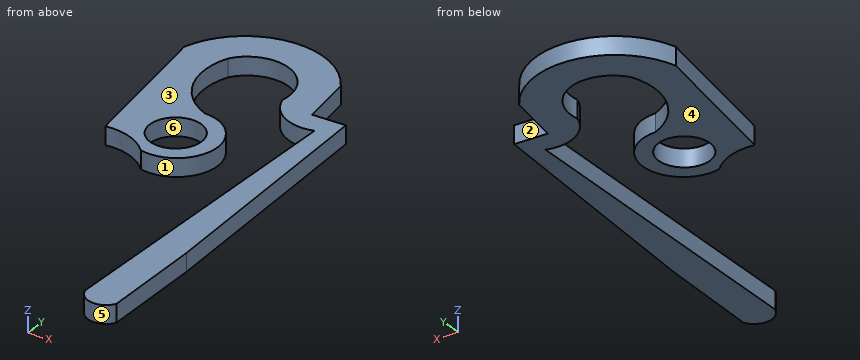
```python
from build123d import *

# Parameters (mm, degrees)
SKETCH1_R           = 1.27
BOSS_EXTRUDE1_DEPTH = 0.889


with BuildPart() as part:
    # Sketch1 → Boss-Extrude1 (new body)
    with BuildSketch(Plane.XY):
        with BuildLine():
            Line((-4.521957117, 7.997023921), (-3.500640843, 0.843746079))
            ThreePointArc((-3.500640843, 0.843746079), (-2.247752793, 0.722417864), (-1.189432305, 0.040943912))
            ThreePointArc((-1.189432305, 0.040943912), (1.231506645, 1.78476828), (-0.761885285, 4.004736172))
            ThreePointArc((-0.761885285, 4.004736172), (-2.523808067, 5.75027928), (-2.507561872, 8.230406029))
            ThreePointArc((-2.507561872, 8.230406029), (-0.008086329, 8.999486055), (1.23243455, 6.697319679))
            ThreePointArc((1.23243455, 6.697319679), (2.203084663, 5.504138097), (3.734868812, 5.364562852))
            Line((3.734868812, 5.364562852), (3.409647754, -10.616831622))
            ThreePointArc((3.409647754, -10.616831622), (4.172569321, -11.302719528), (5.081281403, -10.826553706))
            Line((5.081281403, -10.826553706), (5.081281403, -5.788347659))
            Line((5.081281403, -5.788347659), (4.536062194, 6.463867416))
            Line((4.536062194, 6.463867416), (2.910345816, 6.391523616))
            Line((2.910345816, 6.391523616), (2.548786355, 8.982410145))
            ThreePointArc((2.548786355, 8.982410145), (-1.304965957, 10.774290658), (-4.521957117, 7.997023921))
        make_face()
        with Locations((-0.822961988, 2.012924292)):
            Circle(SKETCH1_R, mode=Mode.SUBTRACT)
    extrude(amount=BOSS_EXTRUDE1_DEPTH)


solid = part.part
```
Input: part model. Units: mm. Frame: model coordinates. Face numbers are marked on the shaded views. A direction names the side the tool comes from. Round coordinates to 2 decimals unless told otherwise and drop trailing zeros. Loops run counter-clockwise (first coordinate to the right, second up) from the corner with the lowest first, then second, coordinate; pieces in that order, holes last. Notation, with made-up numbers: M -13,0.5 L 43,0.5 A23 ccw 43,12.5 Z; hole C 8.25,15 d9. An arc over 180 degrees is marked long. Answer in a Markdown table with one row per item. Add a question column.
1. Ray query, probe 1 along Y at (x, z) = (-1.5, 0.25); probe 2 along Y at (x, z) = (-1.25, 0.05); probe 3 along X at (y, z) = (2, 0.75). Return the intervals inside material, ascending.
2. Section A-A (y = 4.5). Output: boundary loops of the cut face in (x, z), and give its area (3 significant figures).
3. Set-up query: the marked faces 1, 2 and 3. Return all of +Z, -Z, +X, -X, +Y, -Y with unobstructed straight access to the full face (end or side cutting, diameter ignored); none if empty.
4. Section B-B (z = 0.45). Output: boundary loops of the cut face in (x, y).
5. Mould query, pull axis X, two halves, no side actions, for the marked faces 4, 5 and 6. Classes: released by +X, released by -X, zero draft, split by the parting line, or undercut.
6. Section D-D (y = -6.75). Output: boundary loops of the cut face in (x, z), and give its area (3 significant figures).
7. Section C-C (x = -0.25). Output: boundary loops of the cut face in (y, z), and give its area (3 significant figures).
Values follow:
| question | item | result |
|---|---|---|
| 1 | probe 1 | 0.32 to 0.94, 3.09 to 4.42, 9.03 to 10.74 |
| 1 | probe 2 | 0.1 to 0.82, 3.21 to 4.25, 9.1 to 10.78 |
| 1 | probe 3 | -3.67 to -2.09, 0.45 to 1.24, 3.67 to 4.73 |
| 2 | outline | M -4.02,0 L -1.6,0 L -1.6,0.89 L -4.02,0.89 Z; M 3.72,0 L 4.62,0 L 4.62,0.89 L 3.72,0.89 Z |
| 2 | area | 2.96 mm^2 |
| 3 | face 1 | +Z, -Z |
| 3 | face 2 | +Z, -Z, +Y |
| 3 | face 3 | +Z, +X, -X, +Y, -Y |
| 4 | outline | M -4.52,8 L -3.5,0.84 A2.67 cw -1.19,0.04 A2 ccw long -0.76,4 A3.2 cw -2.51,8.23 A2.06 cw 1.23,6.7 A1.98 ccw 3.73,5.36 L 3.41,-10.62 A0.9 ccw 5.08,-10.83 L 5.08,-5.79 L 4.54,6.46 L 2.91,6.39 L 2.55,8.98 A3.92 ccw Z; hole C -0.82,2.01 d2.54 |
| 5 | face 4 | zero draft |
| 5 | face 5 | split by the parting line |
| 5 | face 6 | undercut |
| 6 | outline | M 3.49,0 L 5.08,0 L 5.08,0.89 L 3.49,0.89 Z |
| 6 | area | 1.42 mm^2 |
| 7 | outline | M 0.06,0 L 0.88,0 L 0.88,0.89 L 0.06,0.89 Z; M 3.15,0 L 3.94,0 L 3.94,0.89 L 3.15,0.89 Z; M 9.08,0 L 10.78,0 L 10.78,0.89 L 9.08,0.89 Z |
| 7 | area | 2.94 mm^2 |
